from build123d import *

# Parameters (mm, degrees)
SKETCH_1_R          = 6.1
EXTRUDE_1_DEPTH     = 8.3
SKETCH_2_R          = 4.75
CUT_EXTRUDE_1_DEPTH = 4
SKETCH_3_R          = 3.75
CUT_EXTRUDE_2_DEPTH = 3.5
SKETCH_4_R          = 1.5
CUT_EXTRUDE_3_DEPTH = 4
EXTRUDE_3_DEPTH     = 3
SKETCH_6_R          = 9.011135206
SKETCH_6_R_2        = 6.1
CUT_EXTRUDE_4_DEPTH = 32
SKETCH_7_R          = 0.5
CUT_EXTRUDE_6_DEPTH = 12
SKETCH_8_W          = 2
SKETCH_8_H          = 6.97178126
CUT_EXTRUDE_7_DEPTH = 10
SKETCH_9_W          = 7.844147965
SKETCH_9_H          = 6.877415643
CUT_EXTRUDE_8_DEPTH = 10
SKETCH_10_R         = 0.75
EXTRUDE_4_DEPTH     = 3
SKETCH_11_W         = 15.692438898
SKETCH_11_H         = 2
CUT_EXTRUDE_9_DEPTH = 8


with BuildPart() as part:
    # 草图1 → 凸台-拉伸1 (new body)
    with BuildSketch(Plane(origin=(0, 0, 0), x_dir=(1, 0, 0), z_dir=(0, 1, 0))):
        Circle(SKETCH_1_R)
    extrude(amount=EXTRUDE_1_DEPTH)

    # 草图2 → 切除-拉伸1 (cut)
    with BuildSketch(Plane(origin=(0, 8.3, 0), x_dir=(1, 0, 0), z_dir=(0, 1, 0))):
        Circle(SKETCH_2_R)
    extrude(amount=-CUT_EXTRUDE_1_DEPTH, mode=Mode.SUBTRACT)

    # 草图3 → 切除-拉伸2 (cut)
    with BuildSketch(Plane(origin=(0, 4.3, 0), x_dir=(1, 0, 0), z_dir=(0, 1, 0))):
        Circle(SKETCH_3_R)
    extrude(amount=-CUT_EXTRUDE_2_DEPTH, mode=Mode.SUBTRACT)

    # 草图4 → 切除-拉伸3 (cut)
    with BuildSketch(Plane(origin=(0, 0.8, 0), x_dir=(1, 0, 0), z_dir=(0, 1, 0))):
        Circle(SKETCH_4_R)
    extrude(amount=-CUT_EXTRUDE_3_DEPTH, mode=Mode.SUBTRACT)

    # 草图5 → 凸台-拉伸3 (add, symmetric)
    with BuildSketch(Plane.XY):
        with BuildLine():
            Line((-6.1, 0), (-2.1, 0))
            Line((-2.1, 0), (-2.1, -4.1))
            ThreePointArc((-2.1, -4.1), (-2.656497116, -5.443502884), (-4, -6))
            Line((-4, -6), (-4.2, -6))
            ThreePointArc((-4.2, -6), (-5.543502884, -5.443502884), (-6.1, -4.1))
            Line((-6.1, -4.1), (-6.1, 0))
        make_face()
    extrude(amount=EXTRUDE_3_DEPTH, both=True)

    # 草图6 → 切除-拉伸4 (cut)
    with BuildSketch(Plane(origin=(0, 8.3, 0), x_dir=(1, 0, 0), z_dir=(0, 1, 0))):
        Circle(SKETCH_6_R)
        Circle(SKETCH_6_R_2, mode=Mode.SUBTRACT)
    extrude(amount=-CUT_EXTRUDE_4_DEPTH, mode=Mode.SUBTRACT)

    # 草图7 → 切除-拉伸6 (cut)
    with BuildSketch(Plane.XY.offset(3)):
        with Locations((-4.1, -3.8)):
            Circle(SKETCH_7_R)
    extrude(amount=-CUT_EXTRUDE_6_DEPTH, mode=Mode.SUBTRACT)

    # 草图8 → 切除-拉伸7 (cut)
    with BuildSketch(Plane(origin=(-2.1, 0, 0), x_dir=(0, 0, -1), z_dir=(1, 0, 0))):
        with Locations((0, -3.48589063)):
            Rectangle(SKETCH_8_W, SKETCH_8_H)
    extrude(amount=-CUT_EXTRUDE_7_DEPTH, mode=Mode.SUBTRACT)

    # 草图9 → 切除-拉伸8 (cut)
    with BuildSketch(Plane(origin=(0, 0, -3), x_dir=(-1, 0, 0), z_dir=(0, 0, -1))):
        with Locations((6.022073983, -3.438707822)):
            Rectangle(SKETCH_9_W, SKETCH_9_H)
    extrude(amount=-CUT_EXTRUDE_8_DEPTH, mode=Mode.SUBTRACT)

    # 草图10 → 凸台-拉伸4 (add, symmetric)
    with BuildSketch(Plane.XY):
        with BuildLine():
            Line((-5.1, 0), (5.1, 0))
            Line((5.1, 0), (5.1, -4.5))
            ThreePointArc((5.1, -4.5), (4.074873734, -6.974873734), (1.6, -8))
            Line((1.6, -8), (-1.6, -8))
            ThreePointArc((-1.6, -8), (-4.074873734, -6.974873734), (-5.1, -4.5))
            Line((-5.1, -4.5), (-5.1, 0))
        make_face()
        with Locations((0, -5)):
            Circle(SKETCH_10_R, mode=Mode.SUBTRACT)
    extrude(amount=EXTRUDE_4_DEPTH, both=True)

    # 草图11 → 切除-拉伸9 (cut)
    with BuildSketch(Plane.XZ.offset(8)):
        with Locations((0.217533809, 0)):
            Rectangle(SKETCH_11_W, SKETCH_11_H)
    extrude(amount=-CUT_EXTRUDE_9_DEPTH, mode=Mode.SUBTRACT)


solid = part.part
Could you check a few things on this model? Use its own coordinates, in mm. A direction names the side the tool comes from. Give positions to 0.01 mm unless a question says otherwise; leave off trailing zeros. Loops run counter-clockwise (first coordinate to the right, second up) from the corner with the lowest first, then second, coordinate; pieces in that order, holes last. Notation, with made-up numbers: (77, 59.5) -> (106, 59.5) arc R13 cw to (106, 73.5) -> close; hole circle Ø7 at (46, 83). An arc over 180 degrees is marked (long way). Answer as CSV lines item,"result". Start each with the question number.
(1) Which directions (+Z, -Z, +X, -X, +Y, -Y) give clear straight access to the entire face, cutting with the end or side of a thin tool? Please do faces 1 (the flat face through (5.1, -2, -2)), 2 (the flat face through (0, -4, -1)), 3 (the flat face through (-5.1, -2, -2)), 4 (the cylindrical face through (2.192, 6.328, 4.214)).
(2) If we section it at D-D on y = -5: Write out the boundary of the cut face in (x, z).
(3) I need wall thicknesses on probe 1 along X at (y, z) = (7.2, 0); probe 2 along Y at (x, z) = (0, -2.35); probe 3 along X at (y, z) = (0.6, 0). Which ranges of each line are inside material? Lowest first, please.
(4) I'm going to push flat-ended pins straight in: pin 1 Ø2 at (y, z) = (-1.5, 2) entering from +X; pin 2 Ø6 at (x, y) = (4, 0.5) entering from +Z; pin 3 Ø2 at (x, z) = (-3, 0.5) entering from -Y; pin 4 Ø1.4 at (x, y) = (0, -5) entering from -Z (3 decimals). Where does each tip first touch, or does it pass through?
(5) We'd pull the mould along Y, two halves only. Please class faces 5 (the flat face through (2, 0.8, 0)), 6 (the cylindrical face through (-0.163, -5.732, -2.014)), 7 (the cylindrical face through (-4.05, -7, 2.01)), 8 (the cylindrical face through (-0.163, -5.732, 1.986)): released by +Y, released by -Y, zero draft, split by the parting line, or undercut.
(6) If we section it at C-C on z = 0: Write out the boundary of the cut face in (x, y).
(7) If we section it at B-B on x = 0: Count the separate pieces of the cut face and the enclosed holes in it, then the cut area to 3 significant figures.
(8) If we section it at A-A on y = -0.5: Write out the boundary of the cut face in (x, z).
Computed:
1,face 1,"+Z, -Z, +X, -Y"
1,face 2,"+X, -X, -Y"
1,face 3,"+Z, -Z, -X, -Y"
1,face 4,"+Y"
2,outline,"(-5.06, -3) -> (-0.75, -3) -> (-0.75, -1) -> (-5.06, -1) -> close; (-5.06, 1) -> (-0.75, 1) -> (-0.75, 3) -> (-5.06, 3) -> close; (0.75, -3) -> (5.06, -3) -> (5.06, -1) -> (0.75, -1) -> close; (0.75, 1) -> (5.06, 1) -> (5.06, 3) -> (0.75, 3) -> close"
3,probe 1,"x = -6.1 to -4.75, 4.75 to 6.1"
3,probe 2,"y = -8 to -5.75, -4.25 to 0.8"
3,probe 3,"x = -6.1 to -1.5, 1.5 to 6.1"
4,pin 1,"stops at x = 5.1"
4,pin 2,"stops at z = 6.02"
4,pin 3,"stops at y = -7.96"
4,pin 4,"passes through"
5,face 5,"released by +Y"
5,face 6,"undercut"
5,face 7,"released by -Y"
5,face 8,"undercut"
6,outline,"(-6.1, 0) -> (-1.5, 0) -> (-1.5, 0.8) -> (-3.75, 0.8) -> (-3.75, 4.3) -> (-4.75, 4.3) -> (-4.75, 8.3) -> (-6.1, 8.3) -> close; (1.5, 0) -> (6.1, 0) -> (6.1, 8.3) -> (4.75, 8.3) -> (4.75, 4.3) -> (3.75, 4.3) -> (3.75, 0.8) -> (1.5, 0.8) -> close"
7,separate pieces,"4"
7,enclosed holes,"0"
7,area,"60.6 mm2"
8,outline,"(-5.1, -3) -> (5.1, -3) -> (5.1, -1) -> (-5.1, -1) -> close; (-5.1, 1) -> (5.1, 1) -> (5.1, 3) -> (-5.1, 3) -> close"
